Input: dimensioned drawing with shaded views. Units: mm. Origin: part minimum x, y, z. A direction names the side the tool comes from. Give positions to 0.01 mm unless a question says otherwise; leave off trailing zeros. Write each loop counter-clockwise with the first axis right and the second up, starting at its lowest first coordinate (ties: lowest second). Pieces come first, ordered by that corner, then holes. Notation, with made-up numbers: (86, 20) -> (97, 20) arc R18 cw to (97, 25) -> close; hole circle Ø8 at (12, 52.25). An arc over 180 degrees is marked (long way). Return JSON: item names as keys, results as strings. Group by question number.
Item 1: Section C-C, the plane z = 81. Return loops of the section in (x, y).
Item 2: Section A-A, the plane y = 36. Return loops of the section in (x, z), then the cut area to 3 significant figures.
Item 3: Set-up query: the marked faces 1, 2 and 3. Return all of +Z, -Z, +X, -X, +Y, -Y with unobstructed straight access to the full face (end or side cutting, diameter ignored); none if empty.
Item 4: Pin query (flat end, axial travel): P1, Ø15, axis at x = 20, y = 16.5, coming from the -Z side; P2, Ø6, axis at x = 10.5, y = 17, coming from the +Z side; P3, Ø8, axis at x = 36, z = 68, coming from the +Y side; P4, Ø4, axis at x = 35.5, y = 31.5, coming from the -Z side. Return the tip coordinate at first contact, or that it passes through.
Item 5: Section D-D, the plane y = 14.5. Return loops of the section in (x, z) (1 decimal).
Item 6: Section B-B, the plane x = 25. Return loops of the section in (y, z) (1 decimal), then the cut area to 3 significant figures.
Item 7: Line query: line 1 (Z direction, x = 25, y = 43); line 2 (Z direction, x = 25.5, y = 17.5); line 3 (Y direction, x = 29, z = 32.5) (1 decimal). Output: solid intervals per line, ascending. Write a range as [from, to].
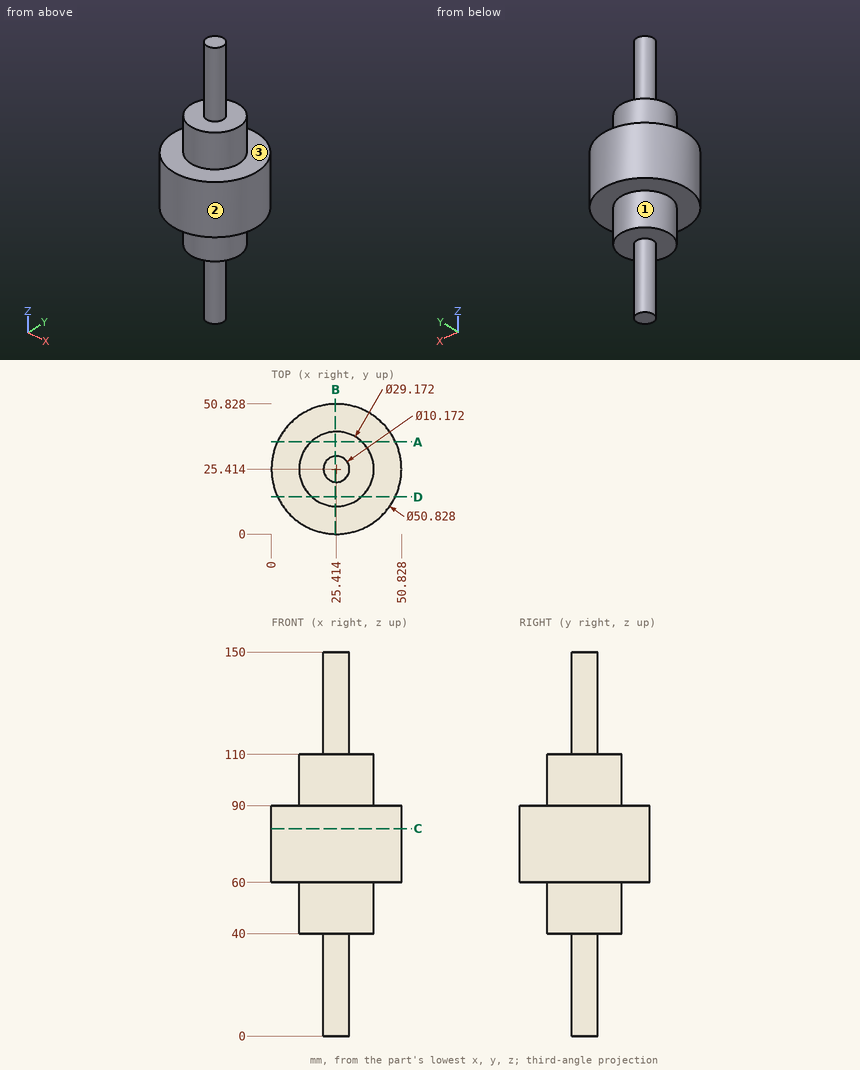
Answer below:
{
 "1": {"outline": "circle Ø50.83 at (25.41, 25.41)"},
 "2": {"outline": "(2.31, 60) -> (15.38, 60) -> (15.38, 40) -> (35.45, 40) -> (35.45, 60) -> (48.52, 60) -> (48.52, 90) -> (35.45, 90) -> (35.45, 110) -> (15.38, 110) -> (15.38, 90) -> (2.31, 90) -> close", "area": "2,190 mm2"},
 "3": {"face 1": "-Z", "face 2": "+Z, -Z", "face 3": "+Z"},
 "4": {"P1": "stops at z = 0", "P2": "stops at z = 110", "P3": "stops at y = 49.96", "P4": "stops at z = 40"},
 "5": {"outline": "(2.5, 60) -> (15.7, 60) -> (15.7, 40) -> (35.1, 40) -> (35.1, 60) -> (48.4, 60) -> (48.4, 90) -> (35.1, 90) -> (35.1, 110) -> (15.7, 110) -> (15.7, 90) -> (2.5, 90) -> close"},
 "6": {"outline": "(0, 60) -> (10.8, 60) -> (10.8, 40) -> (20.3, 40) -> (20.3, 0) -> (30.5, 0) -> (30.5, 40) -> (40, 40) -> (40, 60) -> (50.8, 60) -> (50.8, 90) -> (40, 90) -> (40, 110) -> (30.5, 110) -> (30.5, 150) -> (20.3, 150) -> (20.3, 110) -> (10.8, 110) -> (10.8, 90) -> (0, 90) -> close", "area": "3,500 mm2"},
 "7": {"line 1": "z = [60, 90]", "line 2": "z = [40, 110]", "line 3": "y = [21.8, 29]"}
}
